from build123d import *

# Parameters (mm, degrees)
F1_DEPTH  = 100
F3_DEPTH  = 100.001
F4_W      = 10
F4_H      = 10
F5_DEPTH  = 10.001
F6_DEPTH  = 60.001
F7_W      = 10
F7_H      = 10
F8_DEPTH  = 70.001
F9_W      = 10
F9_H      = 10
F10_DEPTH = 70.001


with BuildPart() as f1:
    # F0 (on Front) → F1 (new body)
    with BuildSketch(Plane.XZ):
        with BuildLine():
            Line((60, -10), (60, 0))
            ThreePointArc((60, 0), (0, 60), (-60, 0))
            Line((-60, 0), (-60, -10))
            Line((-60, -10), (60, -10))
        make_face()
    extrude(amount=F1_DEPTH)

    # F2 (on face) → F3 (cut, through all)
    with BuildSketch(Plane.XZ.offset(100)):
        with BuildLine():
            Line((35, 0), (40, 0))
            ThreePointArc((40, 0), (39.9217985567, 2.5), (39.6875, 4.9902248196))
            ThreePointArc((39.6875, 4.9902248196), (36.3556550657, 3.4232659844), (35, 0))
        make_face()
        with BuildLine():
            ThreePointArc((39.6875, 4.9902248196), (39.9217985567, 2.5), (40, 0))
            Line((40, 0), (35, 0))
            ThreePointArc((35, 0), (40, -5), (45, 0))
            ThreePointArc((45, 0), (43.4232659844, 3.6443449343), (39.6875, 4.9902248196))
        make_face()
        with BuildLine():
            ThreePointArc((35, 0), (36.3556550657, 3.4232659844), (39.6875, 4.9902248196))
            ThreePointArc((39.6875, 4.9902248196), (0, 40), (-39.6875, 4.9902248196))
            ThreePointArc((-39.6875, 4.9902248196), (-36.3556550657, 3.4232659844), (-35, 0))
            Line((-35, 0), (-5, 0))
            ThreePointArc((-5, 0), (0, 5), (5, 0))
            Line((5, 0), (35, 0))
        make_face()
        with BuildLine():
            ThreePointArc((-35, 0), (-36.3556550657, 3.4232659844), (-39.6875, 4.9902248196))
            ThreePointArc((-39.6875, 4.9902248196), (-39.9217985567, 2.5), (-40, 0))
            Line((-40, 0), (-35, 0))
        make_face()
        with BuildLine():
            ThreePointArc((-40, 0), (-39.9217985567, 2.5), (-39.6875, 4.9902248196))
            ThreePointArc((-39.6875, 4.9902248196), (-43.6443449343, -3.4232659844), (-35, 0))
            Line((-35, 0), (-40, 0))
        make_face()
        with BuildLine():
            ThreePointArc((-5, 0), (0, -5), (5, 0))
            Line((5, 0), (-5, 0))
        make_face()
        with BuildLine():
            Line((-5, 0), (5, 0))
            ThreePointArc((5, 0), (0, 5), (-5, 0))
        make_face()
    extrude(amount=-F3_DEPTH, mode=Mode.SUBTRACT)

    # F4 (on Top) → F5 (cut, through all)
    with BuildSketch(Plane.XY):
        with Locations((0, -50)):
            Rectangle(F4_W, F4_H)
    extrude(amount=-F5_DEPTH, mode=Mode.SUBTRACT)

    # F4 (on Top) → F6 (cut, through all)
    with BuildSketch(Plane.XY):
        with Locations((0, -50)):
            Rectangle(F4_W, F4_H)
    extrude(amount=F6_DEPTH, mode=Mode.SUBTRACT)

    # F7 (on face) → F8 (cut, through all)
    with BuildSketch(Plane(origin=(0, 0, -10), x_dir=(1, 0, 0), z_dir=(0, 0, -1))):
        with Locations((45, 50)):
            Rectangle(F7_W, F7_H)
    extrude(amount=-F8_DEPTH, mode=Mode.SUBTRACT)

    # F9 (on face) → F10 (cut, through all)
    with BuildSketch(Plane(origin=(0, 0, -10), x_dir=(1, 0, 0), z_dir=(0, 0, -1))):
        with Locations((-45, 50)):
            Rectangle(F9_W, F9_H)
    extrude(amount=-F10_DEPTH, mode=Mode.SUBTRACT)


solid = f1.part
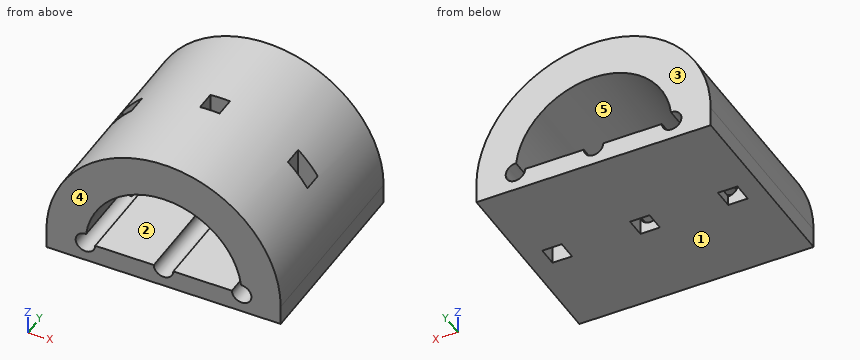
CAD build for the part. Positions are in the model's coordinates, mm. Face numbers are marked on the shaded views. A direction names the side the tool comes from. Coordinates: 2 decimals unless noted, no trailing zeros. Order: outer loops, then holes, each group sorted by start corner. A loop starts at its lowest first (then second) coordinate and runs counter-clockwise, first axis right, second up.
Item 1: Band-saw the part on A-A on z = 28. List the corners of the cut face in (x, y).
Check sheet entries:
outline: (-53.07, -100) - (-28.57, -100) - (-28.57, 0) - (-53.07, 0) - close; (28.57, -100) - (53.07, -100) - (53.07, 0) - (28.57, 0) - close; hole (-50, -55) - (-40, -55) - (-40, -45) - (-50, -45) - close; hole (40, -55) - (50, -55) - (50, -45) - (40, -45) - close
Item 2: Pin check, flat tips, straight feed: pin 1 Ø5 at (y, z) = (-50, 52.5) entering from +X; pin 2 Ø6 at (x, y) = (-42, -70.5) entering from +Z; pin 3 Ø3 at (y, z) = (-48.5, 8.5) entering from -X; pin 4 Ø1 at (x, y) = (42.5, -46) entering from -Z. Stop position of each tip, or through.
Check sheet entries:
pin 1: stops at x = 33.17
pin 2: stops at z = 45.6
pin 3: stops at x = -59.59
pin 4: passes through
Item 3: Band-saw the part on B-B on x = 0. List the corners of the cut face in (y, z).
Check sheet entries:
outline: (-100, -10) - (-55, -10) - (-55, -5) - (-100, -5) - close; (-100, 40) - (-55, 40) - (-55, 60) - (-100, 60) - close; (-45, -10) - (0, -10) - (0, -5) - (-45, -5) - close; (-45, 40) - (0, 40) - (0, 60) - (-45, 60) - close
Item 4: Drill centre lines: L1, parallel to Z at x = -40, y = -75; L2, parallel to Z at x = -0.5, y = -67; L3, parallel to Y at x = -3.5, z = 52. Where is each one in solid material? Low to high.
Check sheet entries:
L1: z = -10 to -5, 5 to 44.72
L2: z = -10 to -4.97, 40 to 60
L3: y = -100 to -55, -45 to 0
Item 5: Band-saw the part on C-C on x = -30.5. List the corners of the cut face in (y, z).
Check sheet entries:
outline: (-100, -10) - (0, -10) - (0, 0) - (-100, 0) - close; (-100, 25.88) - (0, 25.88) - (0, 51.67) - (-100, 51.67) - close
Item 6: Band-saw the part on D-D on y = -92.5. List the corners of the cut face in (x, z), plus the area to 3 significant figures.
Check sheet entries:
outline: (-60, -10) - (60, -10) - (60, 0) arc R60 ccw to (-60, 0) - close; hole (-39.69, 4.99) arc R5 ccw (long way) to (-35, 0) - (-5, 0) arc R5 ccw to (5, 0) - (35, 0) arc R5 ccw (long way) to (39.69, 4.99) arc R40 ccw to start
area: 4,180 mm2
Item 7: 3-axis set-ups, long thin cutter, end or side, ignore diameter. For the marked faces 4 and 5: which of +Z, -Z, +X, -X, +Y, -Y reach the whole face in a straight line?
Check sheet entries:
face 4: +Z, -Z, +X, -X, -Y
face 5: +Y, -Y
Item 8: Two-plate mould, pull along Z, no slides. Class the marked faces 1, 2 and 3: +Z half, -Z half, draft (parallel to the pull), parting line (faces both ways), or undercut.
Check sheet entries:
face 1: -Z half
face 2: undercut
face 3: draft
